```python
from build123d import *

# Parameters (mm, degrees)
SKETCH1_W               = 135.01974
SKETCH1_H               = 146.431289
SKETCH1_R               = 2.5527
BOSS_EXTRUDE1_DEPTH     = 1.6
SKETCH3_W               = 0.5
SKETCH3_H               = 146.431289
CUT_EXTRUDE1_DEPTH      = 1.6
FILLET1_R               = 1
CUT_EXTRUDE2_DEPTH      = 199.847285241
CUT_EXTRUDE2_DEPTH_BACK = 199.847285241
SKETCH4_R               = 1.725


with BuildPart() as part:
    # Sketch1 → Boss-Extrude1 (new body)
    with BuildSketch(Plane.XY):
        with Locations((67.50987, -73.2156445)):
            Rectangle(SKETCH1_W, SKETCH1_H)
        with BuildLine():
            Line((65.489272699, -3.175), (67.6049, -3.175))
            ThreePointArc((67.6049, -3.175), (69.1924, -4.7625), (67.6049, -6.35))
            Line((67.6049, -6.35), (65.489272699, -6.35))
            ThreePointArc((65.489272699, -6.35), (60.7174, -4.7625), (65.489272699, -3.175))
        make_face(mode=Mode.SUBTRACT)
        with Locations((67.50987, -73.2156445)):
            Circle(SKETCH1_R, mode=Mode.SUBTRACT)
        with BuildLine():
            Line((6.094272699, -141.668789), (8.2099, -141.668789))
            ThreePointArc((8.2099, -141.668789), (9.7974, -143.256289), (8.2099, -144.843789))
            Line((8.2099, -144.843789), (6.094272699, -144.843789))
            ThreePointArc((6.094272699, -144.843789), (1.3224, -143.256289), (6.094272699, -141.668789))
        make_face(mode=Mode.SUBTRACT)
        with BuildLine():
            Line((31.494272699, -141.668789), (33.6099, -141.668789))
            ThreePointArc((33.6099, -141.668789), (35.1974, -143.256289), (33.6099, -144.843789))
            Line((33.6099, -144.843789), (31.494272699, -144.843789))
            ThreePointArc((31.494272699, -144.843789), (26.7224, -143.256289), (31.494272699, -141.668789))
        make_face(mode=Mode.SUBTRACT)
        with BuildLine():
            Line((6.094244639, -124.015625), (8.20987194, -124.015625))
            ThreePointArc((8.20987194, -124.015625), (9.79737194, -125.603125), (8.20987194, -127.190625))
            Line((8.20987194, -127.190625), (6.094244639, -127.190625))
            ThreePointArc((6.094244639, -127.190625), (1.32237194, -125.603125), (6.094244639, -124.015625))
        make_face(mode=Mode.SUBTRACT)
        with BuildLine():
            Line((56.894272699, -141.668789), (59.0099, -141.668789))
            ThreePointArc((59.0099, -141.668789), (60.5974, -143.256289), (59.0099, -144.843789))
            Line((59.0099, -144.843789), (56.894272699, -144.843789))
            ThreePointArc((56.894272699, -144.843789), (52.1224, -143.256289), (56.894272699, -141.668789))
        make_face(mode=Mode.SUBTRACT)
        with BuildLine():
            Line((6.094244639, -98.615625), (8.20987194, -98.615625))
            ThreePointArc((8.20987194, -98.615625), (9.79737194, -100.203125), (8.20987194, -101.790625))
            Line((8.20987194, -101.790625), (6.094244639, -101.790625))
            ThreePointArc((6.094244639, -101.790625), (1.32237194, -100.203125), (6.094244639, -98.615625))
        make_face(mode=Mode.SUBTRACT)
        with BuildLine():
            Line((6.094244639, -73.215625), (8.20987194, -73.215625))
            ThreePointArc((8.20987194, -73.215625), (9.79737194, -74.803125), (8.20987194, -76.390625))
            Line((8.20987194, -76.390625), (6.094244639, -76.390625))
            ThreePointArc((6.094244639, -76.390625), (1.32237194, -74.803125), (6.094244639, -73.215625))
        make_face(mode=Mode.SUBTRACT)
        with BuildLine():
            Line((6.094244639, -47.815625), (8.20987194, -47.815625))
            ThreePointArc((8.20987194, -47.815625), (9.79737194, -49.403125), (8.20987194, -50.990625))
            Line((8.20987194, -50.990625), (6.094244639, -50.990625))
            ThreePointArc((6.094244639, -50.990625), (1.32237194, -49.403125), (6.094244639, -47.815625))
        make_face(mode=Mode.SUBTRACT)
        with BuildLine():
            Line((6.094244639, -22.415625), (8.20987194, -22.415625))
            ThreePointArc((8.20987194, -22.415625), (9.79737194, -24.003125), (8.20987194, -25.590625))
            Line((8.20987194, -25.590625), (6.094244639, -25.590625))
            ThreePointArc((6.094244639, -25.590625), (1.32237194, -24.003125), (6.094244639, -22.415625))
        make_face(mode=Mode.SUBTRACT)
        with BuildLine():
            Line((14.689272699, -3.175), (16.8049, -3.175))
            ThreePointArc((16.8049, -3.175), (18.3924, -4.7625), (16.8049, -6.35))
            Line((16.8049, -6.35), (14.689272699, -6.35))
            ThreePointArc((14.689272699, -6.35), (9.9174, -4.7625), (14.689272699, -3.175))
        make_face(mode=Mode.SUBTRACT)
        with BuildLine():
            Line((40.089272699, -3.175), (42.2049, -3.175))
            ThreePointArc((42.2049, -3.175), (43.7924, -4.7625), (42.2049, -6.35))
            Line((42.2049, -6.35), (40.089272699, -6.35))
            ThreePointArc((40.089272699, -6.35), (35.3174, -4.7625), (40.089272699, -3.175))
        make_face(mode=Mode.SUBTRACT)
        with BuildLine():
            Line((118.4049, -6.35), (116.289272699, -6.35))
            ThreePointArc((116.289272699, -6.35), (111.5174, -4.7625), (116.289272699, -3.175))
            Line((116.289272699, -3.175), (118.4049, -3.175))
            ThreePointArc((118.4049, -3.175), (119.9924, -4.7625), (118.4049, -6.35))
        make_face(mode=Mode.SUBTRACT)
        with BuildLine():
            Line((76.20003, -144.843789), (74.084402699, -144.843789))
            ThreePointArc((74.084402699, -144.843789), (69.31253, -143.256289), (74.084402699, -141.668789))
            Line((74.084402699, -141.668789), (76.20003, -141.668789))
            ThreePointArc((76.20003, -141.668789), (77.78753, -143.256289), (76.20003, -144.843789))
        make_face(mode=Mode.SUBTRACT)
        with BuildLine():
            Line((99.484402699, -141.668789), (101.60003, -141.668789))
            ThreePointArc((101.60003, -141.668789), (103.18753, -143.256289), (101.60003, -144.843789))
            Line((101.60003, -144.843789), (99.484402699, -144.843789))
            ThreePointArc((99.484402699, -144.843789), (94.71253, -143.256289), (99.484402699, -141.668789))
        make_face(mode=Mode.SUBTRACT)
        with BuildLine():
            Line((124.884402699, -141.668789), (127.00003, -141.668789))
            ThreePointArc((127.00003, -141.668789), (128.58753, -143.256289), (127.00003, -144.843789))
            Line((127.00003, -144.843789), (124.884402699, -144.843789))
            ThreePointArc((124.884402699, -144.843789), (120.11253, -143.256289), (124.884402699, -141.668789))
        make_face(mode=Mode.SUBTRACT)
        with BuildLine():
            Line((129.919244699, -124.015625), (132.034872, -124.015625))
            ThreePointArc((132.034872, -124.015625), (133.622372, -125.603125), (132.034872, -127.190625))
            Line((132.034872, -127.190625), (129.919244699, -127.190625))
            ThreePointArc((129.919244699, -127.190625), (125.147372, -125.603125), (129.919244699, -124.015625))
        make_face(mode=Mode.SUBTRACT)
        with BuildLine():
            Line((129.919244699, -98.615625), (132.034872, -98.615625))
            ThreePointArc((132.034872, -98.615625), (133.622372, -100.203125), (132.034872, -101.790625))
            Line((132.034872, -101.790625), (129.919244699, -101.790625))
            ThreePointArc((129.919244699, -101.790625), (125.147372, -100.203125), (129.919244699, -98.615625))
        make_face(mode=Mode.SUBTRACT)
        with BuildLine():
            Line((129.919244699, -73.215625), (132.034872, -73.215625))
            ThreePointArc((132.034872, -73.215625), (133.622372, -74.803125), (132.034872, -76.390625))
            Line((132.034872, -76.390625), (129.919244699, -76.390625))
            ThreePointArc((129.919244699, -76.390625), (125.147372, -74.803125), (129.919244699, -73.215625))
        make_face(mode=Mode.SUBTRACT)
        with BuildLine():
            Line((129.919244699, -47.815625), (132.034872, -47.815625))
            ThreePointArc((132.034872, -47.815625), (133.622372, -49.403125), (132.034872, -50.990625))
            Line((132.034872, -50.990625), (129.919244699, -50.990625))
            ThreePointArc((129.919244699, -50.990625), (125.147372, -49.403125), (129.919244699, -47.815625))
        make_face(mode=Mode.SUBTRACT)
        with BuildLine():
            Line((90.889272699, -3.175), (93.0049, -3.175))
            ThreePointArc((93.0049, -3.175), (94.5924, -4.7625), (93.0049, -6.35))
            Line((93.0049, -6.35), (90.889272699, -6.35))
            ThreePointArc((90.889272699, -6.35), (86.1174, -4.7625), (90.889272699, -3.175))
        make_face(mode=Mode.SUBTRACT)
        with BuildLine():
            Line((129.919244699, -22.415625), (132.034872, -22.415625))
            ThreePointArc((132.034872, -22.415625), (133.622372, -24.003125), (132.034872, -25.590625))
            Line((132.034872, -25.590625), (129.919244699, -25.590625))
            ThreePointArc((129.919244699, -25.590625), (125.147372, -24.003125), (129.919244699, -22.415625))
        make_face(mode=Mode.SUBTRACT)
    extrude(amount=BOSS_EXTRUDE1_DEPTH)

    # Sketch3 → Cut-Extrude1 (cut)
    with BuildSketch(Plane.XY.offset(1.6)):
        with Locations((134.76974, -73.2156445)):
            Rectangle(SKETCH3_W, SKETCH3_H)
    extrude(amount=-CUT_EXTRUDE1_DEPTH, mode=Mode.SUBTRACT)

    # Fillet1
    fillet1_edges = [part.edges().sort_by_distance(p)[0] for p in [
        (0, -146.431289, 0.8),
        (0, 0, 0.8),
        (134.51974, 0, 0.8),
        (134.51974, -146.431289, 0.8),
    ]]
    fillet(fillet1_edges, radius=FILLET1_R)

    # Sketch4 → Cut-Extrude2 (cut, two sides: drawn at the far end of the back side and taken through both)
    with BuildSketch(Plane.XY.offset(1.6).offset(-CUT_EXTRUDE2_DEPTH_BACK)):
        with Locations((33.479935, -36.60782225)):
            Circle(SKETCH4_R)
        with Locations((101.539805, -36.60782225)):
            Circle(SKETCH4_R)
        with Locations((101.539805, -109.82346675)):
            Circle(SKETCH4_R)
        with Locations((33.479935, -109.82346675)):
            Circle(SKETCH4_R)
    extrude(amount=CUT_EXTRUDE2_DEPTH + CUT_EXTRUDE2_DEPTH_BACK, mode=Mode.SUBTRACT)


solid = part.part
```
For this review, take the finished solid that the model builds, in its own axes (mm). Coordinates: 2 decimals unless noted, no trailing zeros. Write each loop counter-clockwise with the first axis right and the second up, starting at its lowest first coordinate (ties: lowest second). Pieces come first, ordered by that corner, then holes. Notation, with made-up numbers: (-5, 70) -> (40, 70) arc R23 cw to (40, 78) -> close; hole circle Ø1 at (48, 38). An arc over 180 degrees is marked (long way). Put each result on its own line as item: value.
Q1. Clearance check with a flat-ended pin moving along its axis: pin 1 Ø3 at (x, y) = (71.96, -143.26) entering from -Z. State where the tip first meets the part, or that it passes through.
From the geometry:
pin 1: passes through
Q2. Wall thickness on L1, parallel to X at y = -109.5, z = 0.5; L2, parallel to X at y = -72.5, z = 0.2; L3, parallel to Y at x = 29, z = 0.95: over which ranges is each line inside the solid? List them lowest first.
From the geometry:
L1: x = 0 to 31.79, 35.17 to 99.85, 103.23 to 134.52
L2: x = 0 to 2.66, 5.28 to 65.06, 69.96 to 126.49, 129.11 to 134.52
L3: y = -146.43 to -145.88, -140.63 to 0
Q3. The part is to be moulded in two halves that separate along Y. For faces 1 (the flat face through (51, -72, 1.6)), 2 (the cylindrical face through (33.106, -38.292, 0.789)), say which applies: +Y half, -Y half, draft (parallel to the pull), parting line (faces both ways), or undercut.
From the geometry:
face 1: draft
face 2: undercut
Q4. Take a section at B-B, the plane z = 0.7. Count the separate pieces of the cut face and the enclosed holes in it, then the cut area to 3 significant figures.
From the geometry:
separate pieces: 1
enclosed holes: 26
area: 19,000 mm2
Q5. Take a section at A-A, the plane x = 97.5. State the section outline as (y, z) points.
From the geometry:
outline: (-146.43, 0) -> (-145.9, 0) -> (-145.9, 1.6) -> (-146.43, 1.6) -> close; (-140.61, 0) -> (0, 0) -> (0, 1.6) -> (-140.61, 1.6) -> close
